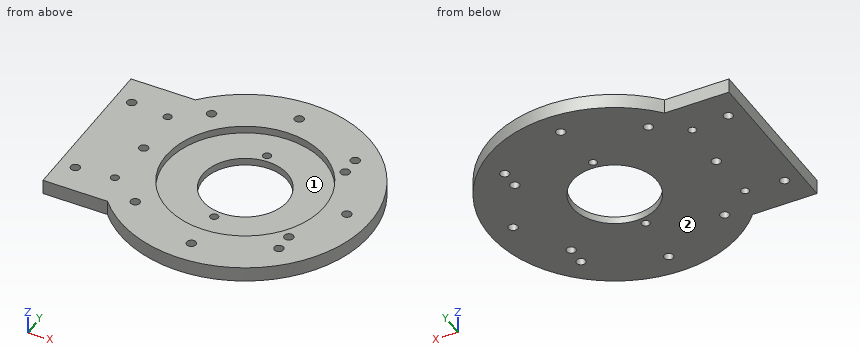
Autodesk Inventor part; units mm, degrees
ref_plane "YZ Plane" through (0, 0, 0) normal (1, 0, 0) x (0, 1, 0)
ref_plane "XZ Plane" through (0, 0, 0) normal (0, 1, 0) x (-1, 0, 0)
ref_plane "XY Plane" through (0, 0, 0) normal (0, 0, 1) x (1, 0, 0)
sketch "スケッチ1" plane through (0, 0, 0) normal (0, 0, 1) x (1, 0, 0)
  line L0 (22.7979, -11.619) -> (22.7979, 11.619) construction
  arc A0 (22.7979, 11.619) -> (11.7979, 16) centre (11.7979, 0) ccw construction
  line L1 (11.7979, 16) -> (-18.2021, 16) construction
  arc A1 (-18.2021, 16) -> (-20.2021, 14) centre (-18.2021, 14) ccw construction
  line L2 (-20.2021, 14) -> (-20.2021, -14) construction
  arc A2 (-20.2021, -14) -> (-18.2021, -16) centre (-18.2021, -14) ccw construction
  line L3 (-18.2021, -16) -> (11.7979, -16) construction
  arc A3 (11.7979, -16) -> (22.7979, -11.619) centre (11.7979, 0) ccw construction
  circle A4 centre (-17.4618, -13.5) radius 1.05 construction
  circle A5 centre (-17.4618, 13.5) radius 1.05 construction
  circle A6 centre (9.5382, -13.5) radius 1.05 construction
  circle A7 centre (9.5382, 13.5) radius 1.05 construction
  circle A8 centre (10.7975, 0) radius 2.7
  circle A9 centre (-57.7021, 15) radius 1.6 construction
  circle A10 centre (-27.7021, 15) radius 1.6 construction
  line L4 (-65.2021, 7.5) -> (-65.2021, 22.5)
  line L5 (-65.2021, 7.5) -> (-20.2021, 7.5) construction
  line L6 (-20.2021, 22.5) -> (-20.2021, 7.5) construction
  line L7 (-65.2021, 22.5) -> (-20.2021, 22.5)
  circle A11 centre (-57.7021, -15) radius 1.6 construction
  circle A12 centre (-27.7021, -15) radius 1.6 construction
  line L8 (-65.2021, -22.5) -> (-65.2021, -7.5)
  line L9 (-65.2021, -22.5) -> (-20.2021, -22.5)
  line L10 (-20.2021, -7.5) -> (-20.2021, -22.5) construction
  line L11 (-65.2021, -7.5) -> (-20.2021, -7.5) construction
  circle A13 centre (-57.7021, -15) radius 1.6 construction
  circle A14 centre (-57.7021, 15) radius 1.6 construction
  line L12 (-50.2021, -22.5) -> (-65.2021, -22.5)
  line L13 (-50.2021, -22.5) -> (-50.2021, 22.5) construction
  line L14 (-65.2021, 22.5) -> (-50.2021, 22.5)
  line L15 (-65.2021, -22.5) -> (-65.2021, 22.5)
  circle A15 centre (10.7975, 0) radius 27.5 construction
  line L16 (-65.2021, 22.5) -> (-14.7118, 22.5)
  line L17 (-65.2021, 22.5) -> (-65.2021, -22.5)
  line L18 (-65.2021, -22.5) -> (-14.7118, -22.5)
  arc A16 (-14.7118, -22.5) -> (-14.7118, 22.5) centre (10.7975, 0) ccw
  circle A17 centre (10.7975, 0) radius 11.5
  circle A18 centre (9.5382, 13.5) radius 1.1
  circle A19 centre (9.5382, -13.5) radius 1.1
  circle A20 centre (-17.4618, 13.5) radius 1.1
  circle A21 centre (-17.4618, -13.5) radius 1.1
  circle A22 centre (-27.7021, 15) radius 1.25
  circle A23 centre (-57.7021, 15) radius 1.25
  circle A24 centre (-57.7021, -15) radius 1.25
  circle A25 centre (-27.7021, -15) radius 1.25
  point P0 (0, 0)
  dimension "d0" = 55
  dimension "d1" = 23
  dimension "d2" = 2.2
  dimension "d3" = 2.2
  dimension "d4" = 2.2
  dimension "d5" = 2.2
  dimension "d6" = 2.5
  dimension "d7" = 2.5
  dimension "d8" = 2.5
  dimension "d9" = 2.5
extrude "押し出し1" add sketch "スケッチ1" along normal blind 4 contours L4 L7 L16 A16 L18 L9 L8 L15
sketch "スケッチ2" plane through (0, 0, 4) normal (0, 0, 1) x (1, 0, 0)
  circle A0 centre (10.7975, 0) radius 11.5
  circle A1 centre (-27.7021, -15) radius 1.25
  circle A2 centre (-57.7021, -15) radius 1.25
  circle A3 centre (-57.7021, 15) radius 1.25
  circle A4 centre (-27.7021, 15) radius 1.25
  circle A5 centre (-17.4618, -13.5) radius 1.1
  circle A6 centre (-17.4618, 13.5) radius 1.1
  circle A7 centre (9.5382, -13.5) radius 1.1
  circle A8 centre (9.5382, 13.5) radius 1.1
  line L0 (-65.2021, 22.5) -> (-65.2021, -22.5)
  line L1 (-65.2021, -22.5) -> (-14.7118, -22.5)
  arc A9 (-14.7118, -22.5) -> (-14.7118, 22.5) centre (10.7975, 0) ccw
  line L2 (-14.7118, 22.5) -> (-65.2021, 22.5)
  circle A10 centre (10.7975, 0) radius 21.5
  point P0 (0, 0)
  dimension "d12" = 43
extrude "押し出し4" cut sketch "スケッチ2" against normal blind 2 contours A10
sketch "スケッチ4" plane through (0, 0, 4) normal (0, 0, 1) x (1, 0, 0)
  circle A0 centre (10.7975, 0) radius 21.5
  circle A1 centre (-27.7021, -15) radius 1.25
  circle A2 centre (-57.7021, -15) radius 1.25
  circle A3 centre (-57.7021, 15) radius 1.25
  circle A4 centre (-27.7021, 15) radius 1.25
  circle A5 centre (-17.4618, -13.5) radius 1.1
  circle A6 centre (-17.4618, 13.5) radius 1.1
  line L0 (-65.2021, 22.5) -> (-65.2021, -22.5)
  line L1 (-65.2021, -22.5) -> (-14.7118, -22.5)
  arc A7 (-14.7118, -22.5) -> (-14.7118, 22.5) centre (10.7975, 0) ccw
  line L2 (-14.7118, 22.5) -> (-65.2021, 22.5)
  circle A8 centre (10.7975, 0) radius 27.6
  circle A9 centre (38.3975, 0) radius 1.25
  circle A10 centre (30.3137, 19.5161) radius 1.25
  circle A11 centre (10.7975, 27.6) radius 1.25
  circle A12 centre (-8.7186, 19.5161) radius 1.25
  circle A13 centre (-16.8025, 0) radius 1.25
  circle A14 centre (-8.7186, -19.5161) radius 1.25
  circle A15 centre (10.7975, -27.6) radius 1.25
  circle A16 centre (30.3137, -19.5161) radius 1.25
  point P0 (0, 0)
  dimension "d25" = 55.2
  dimension "d26" = 2.5
  dimension "d29" = 360
extrude "押し出し5" cut sketch "スケッチ4" against normal through all contours A8 A9 | A8 A9 | A10 A8 | A8 A10 | A16 A8 | A8 A16 | A11 A8 | A8 A11 | A15 A8 | A8 A15 | A12 A8 | A8 A12 | A14 A8 | A8 A14 | A13 A8 | A8 A13
move faces "移動1" translate (33, 0, 0) faces at (-65.2021, 7.5, 1.3333)
sketch "スケッチ8" plane through (0, 0, 0) normal (0, 0, -1) x (-1, 0, 0)
  circle A0 centre (27.7021, -15) radius 1.25
  circle A1 centre (27.7021, 15) radius 1.25
  point P0 (0, 0)
extrude "押し出し7" add sketch "スケッチ8" against normal blind 4
sketch "スケッチ7" plane through (0, 0, 0) normal (0, 0, -1) x (-1, 0, 0)
  circle A0 centre (-30.2979, -14.4) radius 1.6
  circle A1 centre (-30.2979, 14.4) radius 1.6
  circle A2 centre (27.7021, -14.4) radius 1.6
  circle A3 centre (27.7021, 14.4) radius 1.6
  circle A4 centre (-30.2979, -14.4) radius 1.25
  circle A5 centre (-30.2979, 14.4) radius 1.25
  circle A6 centre (27.7021, -14.4) radius 1.25
  circle A7 centre (27.7021, 14.4) radius 1.25
  point P0 (0, 0)
  dimension "d45" = 2.5
  dimension "d46" = 2.5
  dimension "d47" = 2.5
  dimension "d48" = 2.5
extrude "押し出し8" cut sketch "スケッチ7" against normal through all contours A4 | A5 | A6 | A7
properties part number "先端モータマウントC" material "アルミニウム 6061"
Here's how the part is built. I have some questions about the finished solid (model axes, mm). Face numbers are marked on the shaded views. Give positions to 0.01 mm unless a question says otherwise; leave off trailing zeros. Order: outer loops, then holes, each group sorted by start corner. A loop starts at its lowest first (then second) coordinate and runs counter-clockwise, first axis right, second up. Notation, with made-up numbers: (36, 88) -> (63, 88) arc R10 cw to (63, 107) -> close; hole circle Ø8 at (30.25, -32.75). An arc over 180 degrees is marked (long way). One line per item, written item: value. Start each with the question number.
1. Imagine slicing it at A-A, the plane y = 0. List the corners of the cut face in (x, z) for me.
2. I need wall thicknesses on probe 1 along X at (y, z) = (14, 0.35); probe 2 along X at (y, z) = (-13.5, 0.4); probe 3 along Y at (x, z) = (-16.5, 3.65). Which ranges of each line are inside material? Lowest first, please. Write a range as from..to.
3. Imagine slicing it at D-D, the plane x = 25. List the corners of the cut face in (y, z) for me, plus the area to 3 significant figures.
4. Imagine slicing it at B-B, the plane z = 0.9. Count the separate pieces of the cut face and the enclosed holes in it, plus the area to 3 significant figures.
5. We'd pull the mould along X, two halves only. Please class the marked faces 1 and 2: released by +X, released by -X, zero draft, split by the parting line, or undercut.
6. Imagine slicing it at C-C, the plane y = 27.6. List the corners of the cut face in (x, z) for me, plus the area to 3 significant figures.
7. Will these pins go through, and if not, where does the flat tip stop? pin 1 Ø2 at (x, z) = (27, 1.5) entering from -Y; pin 2 Ø1.2 at (x, z) = (-25.5, 2) entering from +Y; pin 3 Ø3 at (x, y) = (9.54, -13.5) entering from +Z.
Values follow:
1. outline: (-32.2, 0) -> (-18.05, 0) -> (-18.05, 4) -> (-32.2, 4) -> close; (-15.55, 0) -> (-0.7, 0) -> (-0.7, 2) -> (-10.7, 2) -> (-10.7, 4) -> (-15.55, 4) -> close; (22.3, 0) -> (37.15, 0) -> (37.15, 4) -> (32.3, 4) -> (32.3, 2) -> (22.3, 2) -> close; (39.65, 0) -> (44.81, 0) -> (44.81, 4) -> (39.65, 4) -> close
2. probe 1: x = -32.2..-28.89, -26.52..-18.44, -16.48..8.56, 10.52..29.11, 31.48..41.8
2. probe 2: x = -32.2..-28.57, -26.83..-18.56, -16.36..8.44, 10.64..29.43, 31.17..42.02
2. probe 3: y = -22.5..-14.03, -12.97..-1.21, 1.21..12.97, 14.03..22.5
3. outline: (-30.91, 0) -> (30.91, 0) -> (30.91, 4) -> (16.14, 4) -> (16.14, 2) -> (-16.14, 2) -> (-16.14, 4) -> (-30.91, 4) -> close
3. area: 183 mm2
4. separate pieces: 1
4. enclosed holes: 17
4. area: 3,670 mm2
5. face 1: undercut
5. face 2: zero draft
6. outline: (-9.08, 0) -> (9.55, 0) -> (9.55, 4) -> (-9.08, 4) -> close; (12.05, 0) -> (30.68, 0) -> (30.68, 4) -> (12.05, 4) -> close
6. area: 149 mm2
7. pin 1: stops at y = -30.43
7. pin 2: stops at y = 22.5
7. pin 3: stops at z = 2
